CAD build for the part. Positions are in the model's coordinates, mm. A direction names the side the tool comes from. Coordinates: 2 decimals unless noted, no trailing zeros. Loops run counter-clockwise (first coordinate to the right, second up) from the corner with the lowest first, then second, coordinate; pieces in that order, holes last.
1) Saw through at A-A, the plane y = 0. Write the cut outline in (x, z) (3 decimals), and give its area (3 significant figures).
2) Pin check, flat tips, straight feed: pin 1 Ø3 at (x, y) = (2.5, 0.5) entering from +Z (3 decimals); pin 2 Ø2 at (x, y) = (2, -3) entering from +Z; pin 3 Ø2 at (x, z) = (14, 0) entering from -Y (3 decimals). Stop position of each tip, or through.
3) Wall check: line 1 along Y through (x, z) = (11.5, 0) (3 decimals); line 2 along X through (y, z) = (3.5, 0.25). Give the ranges that are in metal, low to high.
4) Two-plate mould, pull along Z, no slides. Class faces 1 (the flat face through (-1.493, -2.436, 1.38)), 2 (the flat face through (0, -3, 2)), 3 (the cylindrical face through (-0.99, 4.46, -0.59)): +Z half, -Z half, draft (parallel to the pull), parting line (faces both ways), or undercut.
5) Which spindle directions (+Z, -Z, +X, -X, +Y, -Y) get a long thin tool onto all of the face, cutting with end or side? Do faces 4 (the flat face through (-1.493, 2.414, 1.42)), 5 (the flat face through (-2, 0, 3)), 6 (the cylindrical face through (2.12, -3.1, 0.69)), 7 (the cylindrical face through (11.98, -3.1, 0.69)), 8 (the cylindrical face through (7.45, 0.07, -1.5)). Say none if no direction does.
6) Saw through at B-B, the plane y = 4. Write the cut outline in (x, z).
```python
from build123d import *

# Parameters (mm, degrees)
SKETCH1_R                     = 3.175
BOSS_EXTRUDE1_DEPTH           = 18
SKETCH4_R                     = 4.5
BOSS_EXTRUDE2_DEPTH           = 2
BOSS_EXTRUDE3_START           = -6.3
SKETCH4_3_R                   = 4.5
BOSS_EXTRUDE3_DEPTH           = 2
CUT_EXTRUDE3_DEPTH            = 21.988091862
CUT_EXTRUDE3_DEPTH_BACK       = 21.988091862
SKETCH5_R                     = 1.5
CUT_EXTRUDE4_DEPTH            = 21.988091862
CUT_EXTRUDE4_DEPTH_BACK       = 1
CSK_FOR_M3_SFHCS1_D           = 3
CSK_FOR_M3_SFHCS1_DEPTH       = 5.098709071
CSK_FOR_M3_SFHCS1_CSINK_D     = 6.72
CSK_FOR_M3_SFHCS1_CSINK_ANGLE = 90
CSK_FOR_M3_SFHCS1_TIP         = 0.901290929


with BuildPart() as part:
    # Sketch1 → Boss-Extrude1 (new body)
    with BuildSketch(Plane(origin=(0, 0, 0), x_dir=(0, 0, -1), z_dir=(1, 0, 0))):
        Circle(SKETCH1_R)
    extrude(amount=BOSS_EXTRUDE1_DEPTH)

    # Sketch4 → Boss-Extrude2 (add)
    with BuildSketch(Plane.ZY):
        Circle(SKETCH4_R)
    extrude(amount=BOSS_EXTRUDE2_DEPTH)

    # Sketch4<3> → Boss-Extrude3 (add)
    with BuildSketch(Plane.ZY.offset(BOSS_EXTRUDE3_START)):
        Circle(SKETCH4_3_R)
    extrude(amount=BOSS_EXTRUDE3_DEPTH)

    # Sketch5 → Cut-Extrude3 (cut, two sides: drawn at the far end of the back side and taken through both)
    with BuildSketch(Plane.ZY.offset(2).offset(-CUT_EXTRUDE3_DEPTH_BACK)):
        Circle(SKETCH5_R)
    extrude(amount=CUT_EXTRUDE3_DEPTH + CUT_EXTRUDE3_DEPTH_BACK, mode=Mode.SUBTRACT)

    # Sketch6 → Cut-Extrude4 (cut, two sides: drawn at the far end of the back side and taken through both)
    with BuildSketch(Plane.ZY.offset(2).offset(-CUT_EXTRUDE4_DEPTH_BACK)):
        Polygon((2.8, -1.616580754), (2.8, 1.616580754), (0, 3.233161507), (-2.8, 1.616580754), (-2.8, -1.616580754), (0, -3.233161507), align=None)
    extrude(amount=CUT_EXTRUDE4_DEPTH + CUT_EXTRUDE4_DEPTH_BACK, mode=Mode.SUBTRACT)

    # CSK for M3 SFHCS1
    with Locations(Plane(origin=(18, 0, 0), x_dir=(0, 0, -1), z_dir=(1, 0, 0))):
        with Locations((0, 0)):
            CounterSinkHole(CSK_FOR_M3_SFHCS1_D / 2, CSK_FOR_M3_SFHCS1_CSINK_D / 2, depth=CSK_FOR_M3_SFHCS1_DEPTH, counter_sink_angle=CSK_FOR_M3_SFHCS1_CSINK_ANGLE)
            with Locations((0, 0, -(CSK_FOR_M3_SFHCS1_DEPTH + CSK_FOR_M3_SFHCS1_TIP / 2))):  # 118° drill point
                Cone(0, CSK_FOR_M3_SFHCS1_D / 2, CSK_FOR_M3_SFHCS1_TIP, mode=Mode.SUBTRACT)


solid = part.part
```
Data:
1. outline: (-2, -4.5) - (0, -4.5) - (0, -3.175) - (4.3, -3.175) - (4.3, -4.5) - (6.3, -4.5) - (6.3, -3.175) - (17.815, -3.175) - (16.14, -1.5) - (-1, -1.5) - (-1, -2.8) - (-2, -2.8) - close; (-2, 2.8) - (-1, 2.8) - (-1, 1.5) - (16.14, 1.5) - (17.815, 3.175) - (6.3, 3.175) - (6.3, 4.5) - (4.3, 4.5) - (4.3, 3.175) - (0, 3.175) - (0, 4.5) - (-2, 4.5) - close
1. area: 71.6 mm2
2. pin 1: stops at z = 3.175
2. pin 2: stops at z = 2.47
2. pin 3: stops at y = -3.175
3. line 1: y = -3.175 to -1.5, 1.5 to 3.175
3. line 2: x = -2 to 0, 4.3 to 6.3
4. face 1: undercut
4. face 2: draft
4. face 3: parting line
5. face 4: -X
5. face 5: +Z, -Z, -X, +Y, -Y
5. face 6: none
5. face 7: +X
5. face 8: +X, -X
6. outline: (-2, -2.06) - (0, -2.06) - (0, 2.06) - (-2, 2.06) - close; (4.3, -2.06) - (6.3, -2.06) - (6.3, 2.06) - (4.3, 2.06) - close
